Geometry: final body of the model. Coordinates: model frame, mm. Face numbers are marked on the shaded views. Round coordinates to 2 decimals unless told otherwise and drop trailing zeros. Loops run counter-clockwise (first coordinate to the right, second up) from the corner with the lowest first, then second, coordinate; pieces in that order, holes last. Notation, with made-up numbers: (-25, 60.5) - (-16, 60.5) arc R31 ccw to (-16, 99.5) - close; hole circle Ø7 at (19.25, 67.25). An arc over 180 degrees is marked (long way). Write item = value, one per line. Start each with the question number.
Item 1: Section B-B (z = 5.5). Return loops of the section in (x, y).
Item 2: Draft query along X for the marked faces 1 and 2. Return one class per face: pulls with the +X half, pulls with the -X half, needs draft (parallel to the pull), parting line crosses it, or undercut.
Item 3: Section D-D (x = 16.5). Return loops of the section in (y, z).
Item 4: First-contact query: pin 1 (2.5 mm diameter, centred on x = 33, y = 14.5, fed in from +Z); pin 2 (3.5 mm diameter, centred on x = -33, y = 17, fed in from -Z); pin 3 (1.7 mm diameter, centred on x = 33, y = 5.5, fed in from +Z); pin 4 (2 mm diameter, centred on y = 18.47, z = 20.04, fed in from -X). Flat tips, straight axial feed; report the tip coordinate or a pass-through.
Item 5: Section A-A (y = 12.75). Return loops of the section in (x, z).
Item 6: Section C-C (x = 30.5). Return loops of the section in (y, z), plus the area to 3 significant figures.
Item 7: Line query: line 1 (X direction, y = 11, z = -19.5); line 2 (X direction, y = 1.5, z = 37) (1 decimal); line 3 (Z direction, x = 18, y = 3.25). Output: solid intervals per line, ascending. Write a range as from..to.
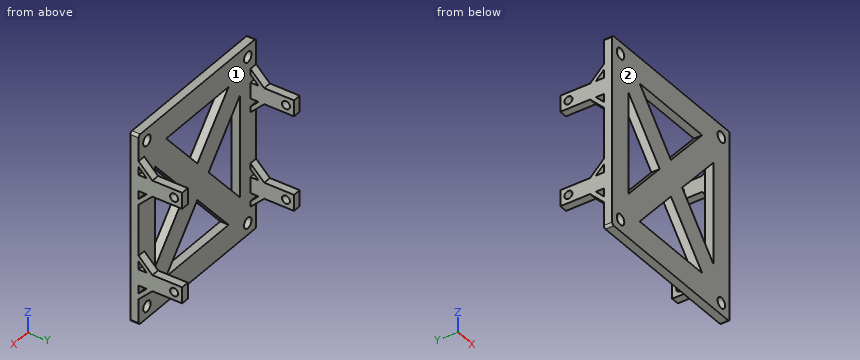
from build123d import *

# Parameters (mm, degrees)
SKETCH1_W                                  = 70.427
SKETCH1_H                                  = 60.325
BOSS_EXTRUDE1_DEPTH                        = 3.5
SKETCH4_R                                  = 1.7
BOSS_EXTRUDE2_DEPTH                        = 3.4
MIRROR1_AT_THE_SECOND_PLANE_COPY_1_SKETC_R = 1.7
MIRROR1_AT_THE_SECOND_PLANE_COPY_1_DEPTH   = 3.4
SKETCH6_W                                  = 70.427
SKETCH6_H                                  = 10
SKETCH6_R                                  = 2.25
BOSS_EXTRUDE3_DEPTH                        = 3.5
FILLET1_R                                  = 1
CUT_EXTRUDE3_DEPTH                         = 19.368750112
CUT_EXTRUDE3_DEPTH_BACK                    = 4.5


with BuildPart() as part:
    # Sketch1 → Boss-Extrude1 (new body)
    with BuildSketch(Plane(origin=(0, 0, 0), x_dir=(1, 0, 0), z_dir=(0, 1, 0))):
        Rectangle(SKETCH1_W, SKETCH1_H)
    extrude(amount=BOSS_EXTRUDE1_DEPTH)

    # Sketch4 → Boss-Extrude2 (add)
    with BuildSketch(Plane.ZY.offset(35.2135)):
        Polygon((-29.239788056, 3.5), (-23.435625, 9.304163056), (-23.435625, 21.868750112), (-16.635625, 21.868750112), (-16.635625, 9.304163056), (-10.831461944, 3.5), (-13.235625, 3.5), (-16.635625, 6.9), (-16.635625, 3.5), (-23.435625, 3.5), (-23.435625, 6.9), (-26.835625, 3.5), align=None)
        with Locations((-20.035625, 18.468750112)):
            Circle(SKETCH4_R, mode=Mode.SUBTRACT)
    boss_extrude2 = extrude(amount=-BOSS_EXTRUDE2_DEPTH)

    # Mirror1: Boss-Extrude2 across plane
    add(boss_extrude2.mirror(Plane(origin=(0, 0, 0), x_dir=(0, 0, 1), z_dir=(1, 0, 0))))

    # Mirror1 at the second plane: Boss-Extrude2 across plane
    add(boss_extrude2.mirror(Plane(origin=(0, 0, 0), x_dir=(1, 0, 0), z_dir=(0, 0, -1))))

    # Mirror1 at the second plane copy 1 sketc → Mirror1 at the second plane copy 1 (add)
    with BuildSketch(Plane(origin=(35.2135, 0, 0), x_dir=(0, 0, -1), z_dir=(1, 0, 0))):
        Polygon((-29.239788056, 3.5), (-23.435625, 9.304163056), (-23.435625, 21.868750112), (-16.635625, 21.868750112), (-16.635625, 9.304163056), (-10.831461944, 3.5), (-13.235625, 3.5), (-16.635625, 6.9), (-16.635625, 3.5), (-23.435625, 3.5), (-23.435625, 6.9), (-26.835625, 3.5), align=None)
        with Locations((-20.035625, 18.468750112)):
            Circle(MIRROR1_AT_THE_SECOND_PLANE_COPY_1_SKETC_R, mode=Mode.SUBTRACT)
    extrude(amount=-MIRROR1_AT_THE_SECOND_PLANE_COPY_1_DEPTH)

    # Sketch6 → Boss-Extrude3 (add)
    with BuildSketch(Plane(origin=(0, 3.5, 0), x_dir=(1, 0, 0), z_dir=(0, 1, 0))):
        with Locations((0, 35.1625)):
            Rectangle(SKETCH6_W, SKETCH6_H)
        with Locations((-30.2135, 35.1625)):
            Circle(SKETCH6_R, mode=Mode.SUBTRACT)
        with Locations((30.2135, 35.1625)):
            Circle(SKETCH6_R, mode=Mode.SUBTRACT)
    boss_extrude3 = extrude(amount=-BOSS_EXTRUDE3_DEPTH)

    # Mirror2: Boss-Extrude3 across plane
    add(boss_extrude3.mirror(Plane.XY))

    # Fillet1
    fillet1_edges = [part.edges().sort_by_distance(p)[0] for p in [
        (-35.2135, 1.75, -40.1625),
        (35.2135, 1.75, -40.1625),
        (-35.2135, 1.75, 40.1625),
        (35.2135, 1.75, 40.1625),
    ]]
    fillet(fillet1_edges, radius=FILLET1_R)

    # Sketch7 → Cut-Extrude3 (cut, two sides)
    with BuildSketch(Plane(origin=(0, 3.5, 0), x_dir=(1, 0, 0), z_dir=(0, 1, 0))) as cut_extrude3_sk:
        Polygon((0, 7.735286309), (18.727217831, 29.239788056), (-18.727217831, 29.239788056), align=None)
        Polygon((25.4635, -21.504501748), (25.4635, 21.504501748), (6.736282169, 0), align=None)
        Polygon((-18.727217831, -29.239788056), (18.727217831, -29.239788056), (0, -7.735286309), align=None)
        Polygon((-6.736282169, 0), (-25.4635, 21.504501748), (-25.4635, -21.504501748), align=None)
    extrude(amount=CUT_EXTRUDE3_DEPTH, mode=Mode.SUBTRACT)
    extrude(cut_extrude3_sk.sketch, amount=-CUT_EXTRUDE3_DEPTH_BACK, mode=Mode.SUBTRACT)


solid = part.part
Taken from the geometry:
q1.outline = (-35.21, 0) - (-25.46, 0) - (-25.46, 3.5) - (-35.21, 3.5) - close; (-11.53, 0) - (11.53, 0) - (11.53, 3.5) - (-11.53, 3.5) - close; (25.46, 0) - (35.21, 0) - (35.21, 3.5) - (25.46, 3.5) - close
q2.face_1 = undercut
q2.face_2 = needs draft
q3.outline = (0, -40.16) - (3.5, -40.16) - (3.5, -29.24) - (0, -29.24) - close; (0, -26.68) - (3.5, -26.68) - (3.5, -11.21) - (0, -11.21) - close; (0, 11.21) - (3.5, 11.21) - (3.5, 26.68) - (0, 26.68) - close; (0, 29.24) - (3.5, 29.24) - (3.5, 40.16) - (0, 40.16) - close
q4.pin_1 = 23.44
q4.pin_2 = -23.44
q4.pin_3 = 28.09
q4.pin_4 = through
q5.outline = (-35.21, -23.44) - (-31.81, -23.44) - (-31.81, -16.64) - (-35.21, -16.64) - close; (-35.21, 16.64) - (-31.81, 16.64) - (-31.81, 23.44) - (-35.21, 23.44) - close; (31.81, -23.44) - (35.21, -23.44) - (35.21, -16.64) - (31.81, -16.64) - close; (31.81, 16.64) - (35.21, 16.64) - (35.21, 23.44) - (31.81, 23.44) - close
q6.outline = (0, -40.16) - (3.5, -40.16) - (3.5, -37.39) - (0, -37.39) - close; (0, -32.93) - (3.5, -32.93) - (3.5, 32.93) - (0, 32.93) - close; (0, 37.39) - (3.5, 37.39) - (3.5, 40.16) - (0, 40.16) - close
q6.area = 250 mm^2
q7.line_1 = -35.21..-31.81, 31.81..35.21
q7.line_2 = -35.2..-31.5, -28.9..28.9, 31.5..35.2
q7.line_3 = -40.16..-29.24, -28.4..-12.93, 12.93..28.4, 29.24..40.16
